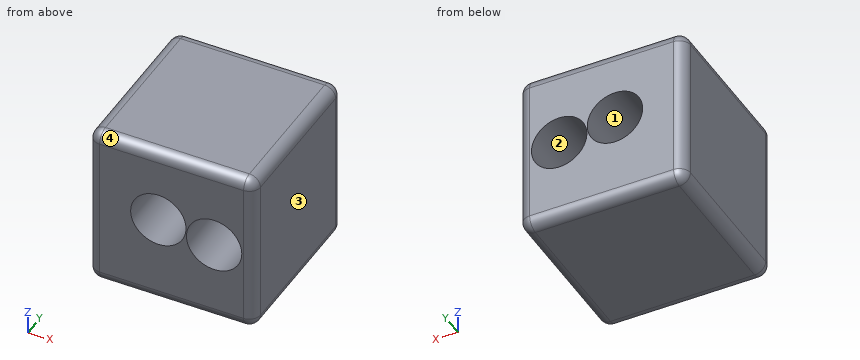
from build123d import *

# Parameters (mm, degrees)
F0_W     = 76.2
F0_H     = 76.2
F1_DEPTH = 76.2
F2_R     = 5.08
F4_D     = 25.4
F6_D     = 25.4


with BuildPart() as f1:
    # F0 (on Front) → F1 (new body)
    with BuildSketch(Plane.XZ):
        with Locations((6.111342, -3.729404)):
            Rectangle(F0_W, F0_H)
    extrude(amount=F1_DEPTH)

    # F2
    f2_edges = [f1.edges().sort_by_distance(p)[0] for p in [
        (44.211342, -38.1, 34.370596),
        (6.111342, -76.2, 34.370596),
        (44.211342, -76.2, -3.729404),
        (44.211342, -38.1, -41.829404),
        (6.111342, -76.2, -41.829404),
        (-31.988658, -38.1, 34.370596),
        (6.111342, 0, 34.370596),
        (44.211342, 0, -3.729404),
        (6.111342, 0, -41.829404),
        (-31.988658, -38.1, -41.829404),
        (-31.988658, 0, -3.729404),
        (-31.988658, -76.2, -3.729404),
    ]]
    fillet(f2_edges, radius=F2_R)

    # F4 (through all)
    with Locations(Plane.XZ.offset(76.2)):
        with Locations((0, 0)):
            Hole(F4_D / 2)

    # F6 (through all)
    with Locations(Plane(origin=(0, 0, 0), x_dir=(-1, 0, 0), z_dir=(0, 1, 0))):
        with Locations((-25.59245, -3.729404)):
            Hole(F6_D / 2)


solid = f1.part
Geometry: final body of the model. Coordinates: model frame, mm. Face numbers are marked on the shaded views. Give positions to 0.01 mm unless a question says otherwise; leave off trailing zeros. Loops run counter-clockwise (first coordinate to the right, second up) from the corner with the lowest first, then second, coordinate; pieces in that order, holes last. Notation, with made-up numbers: (47.5, -4.5) - (64.5, -4.5) arc R22 cw to (64.5, 25.5) - close; hole circle Ø6 at (38.5, 59.5). An arc over 180 degrees is marked (long way). Answer as CSV lines item,"result". Start each with the question number.
1. Section A-A, the plane x = 9. Return loops of the section in (y, z).
2. Section B-B, the plane z = -9.5. Return loops of the section in (x, y), plus the area to 3 significant figures.
3. Ray query, L1, parallel to X at y = -61, z = 4; L2, parallel to Z at x = 0, y = -10; L3, parallel to X at y = -19.5, z = -9. Return the intervals inside material, ascending.
4. Section D-D, the plane z = 10.5. Return loops of the section in (x, y), plus the area to 3 significant figures.
5. Draft query along Z for the marked faces 1, 2, 3 and 4. Return one class per face: released by +Z, released by -Z, zero draft, split by the parting line, or undercut.
6. Section C-C, the plane y = -33. Return loops of the section in (x, z).
Answers:
1,outline,"(-76.2, -36.75) arc R5.08 ccw to (-71.12, -41.83) - (-5.08, -41.83) arc R5.08 ccw to (0, -36.75) - (0, -8.96) - (-76.2, -8.96) - close; (-76.2, 8.96) - (0, 8.96) - (0, 29.29) arc R5.08 ccw to (-5.08, 34.37) - (-71.12, 34.37) arc R5.08 ccw to (-76.2, 29.29) - close"
2,outline,"(-31.99, -71.12) arc R5.08 ccw to (-26.91, -76.2) - (-8.43, -76.2) - (-8.43, 0) - (-26.91, 0) arc R5.08 ccw to (-31.99, -5.08) - close; (8.43, -76.2) - (14.28, -76.2) - (14.28, 0) - (8.43, 0) - close; (36.91, -76.2) - (39.13, -76.2) arc R5.08 ccw to (44.21, -71.12) - (44.21, -5.08) arc R5.08 ccw to (39.13, 0) - (36.91, 0) - close"
2,area,"2,780 mm2"
3,L1,"x = -31.99 to -12.05, 12.05 to 15.52, 35.67 to 44.21"
3,L2,"z = -41.83 to -12.7, 12.7 to 34.37"
3,L3,"x = -31.99 to -8.96, 8.96 to 14.04, 37.15 to 44.21"
4,outline,"(-31.99, -71.12) arc R5.08 ccw to (-26.91, -76.2) - (-7.14, -76.2) - (-7.14, 0) - (-26.91, 0) arc R5.08 ccw to (-31.99, -5.08) - close; (7.14, -76.2) - (39.13, -76.2) arc R5.08 ccw to (44.21, -71.12) - (44.21, -5.08) arc R5.08 ccw to (39.13, 0) - (7.14, 0) - close"
4,area,"4,700 mm2"
5,face 1,"undercut"
5,face 2,"undercut"
5,face 3,"zero draft"
5,face 4,"released by +Z"
6,outline,"(-31.99, -36.75) arc R5.08 ccw to (-26.91, -41.83) - (39.13, -41.83) arc R5.08 ccw to (44.21, -36.75) - (44.21, 29.29) arc R5.08 ccw to (39.13, 34.37) - (-26.91, 34.37) arc R5.08 ccw to (-31.99, 29.29) - close; hole circle Ø25.4 at (0, 0); hole circle Ø25.4 at (25.59, -3.73)"
